Job drawing, mm, ordinate dimensions from the low corner. One solid piece. A direction names the side the tool comes from. Give positions to 0.01 mm unless a question says otherwise; leave off trailing zeros. Write each loop counter-clockwise with the first axis right and the second up, starting at its lowest first coordinate (ties: lowest second). Pieces come first, ordered by that corner, then holes. Notation, with made-up numbers: (-8.75, 83) - (44.25, 83) arc R36 ccw to (44.25, 122) - close; hole circle Ø10 at (0, -37.5). An arc over 180 degrees is marked (long way). Answer as a JSON object with one key per item and string values.
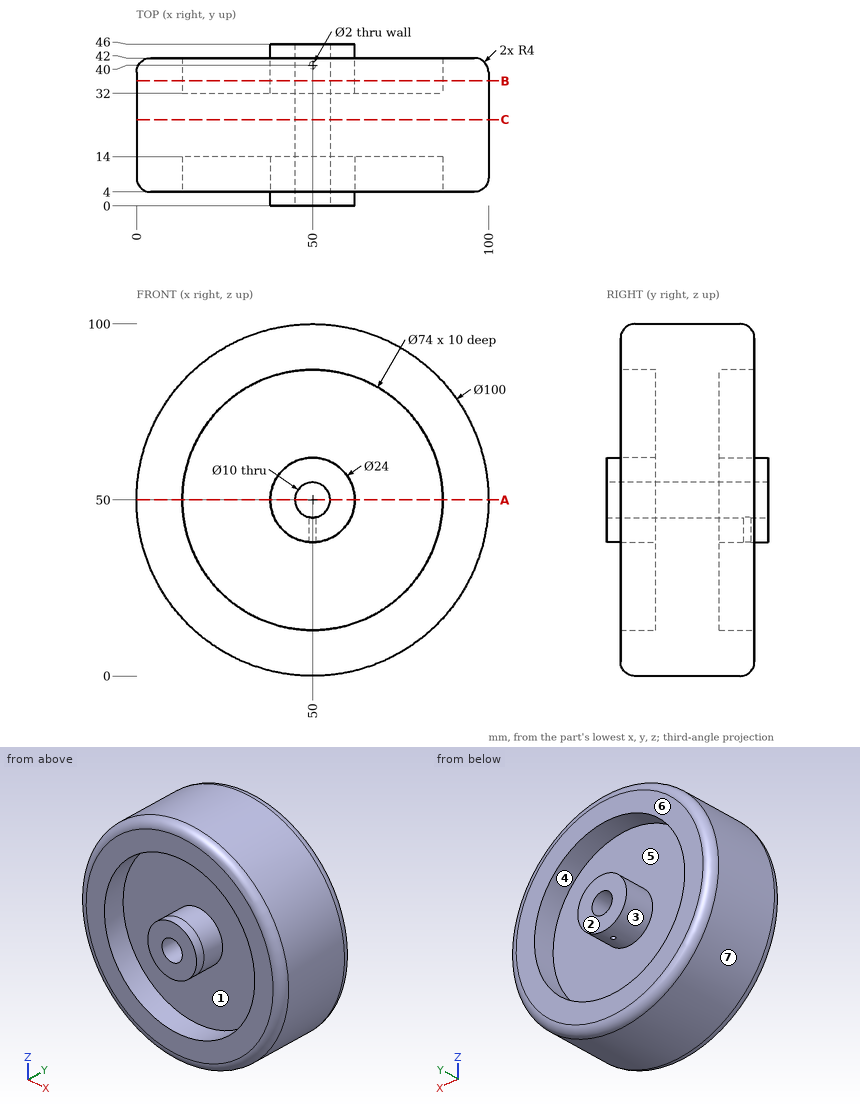
Item 1: Flat gauge pins, fed straight in: P1, Ø12, axis at x = 76.5, z = 62.5, coming from the -Y side; P2, Ø1.5, axis at x = 89, z = 57, coming from the -Y side; P3, Ø3, axis at x = 50, y = 40, coming from the -Z side. Where does each tip first touch, or does it go through?
Entries:
{"P1": "y = 14", "P2": "y = 4", "P3": "z = 0.03"}
Item 2: Probe line 1 (X direction, y = 8.5, z = 50); line 2 (Z direction, x = 53.5, y = 37.5); line 3 (X direction, y = 7, z = 50). List the from-to ranges inside material, lowest first. Write a range as from..to.
Entries:
{"line 1": "0..13, 38..45, 55..62, 87..100", "line 2": "0.12..13.17, 38.52..46.43, 53.57..61.48, 86.83..99.88", "line 3": "0.13..13, 38..45, 55..62, 87..99.87"}
Item 3: Mould opens along Z. For the marked faces 4, 5, 6 and 7 say: +Z half, -Z half, draft (parallel to the pull), parting line (faces both ways), or undercut.
Entries:
{"face 4": "undercut", "face 5": "undercut", "face 6": "draft", "face 7": "parting line"}
Item 4: Cut at B-B (y = 35.5). Give the cut face in (x, z), and give its area (3 significant figures).
Entries:
{"outline": "circle Ø100 at (50, 50); circle Ø24 at (50, 50); hole circle Ø74 at (50, 50); hole circle Ø10 at (50, 50)", "area": "3,930 mm2"}
Item 5: Cut at A-A (z = 50). Give the cut face in (x, y), and give its area (3 significant figures).
Entries:
{"outline": "(0, 8) arc R4 ccw to (4, 4) - (13, 4) - (13, 14) - (38, 14) - (38, 0) - (45, 0) - (45, 46) - (38, 46) - (38, 32) - (13, 32) - (13, 42) - (4, 42) arc R4 ccw to (0, 38) - close; (55, 0) - (62, 0) - (62, 14) - (87, 14) - (87, 4) - (96, 4) arc R4 ccw to (100, 8) - (100, 38) arc R4 ccw to (96, 42) - (87, 42) - (87, 32) - (62, 32) - (62, 46) - (55, 46) - close", "area": "2,520 mm2"}
Item 6: Which spindle directions (+Z, -Z, +X, -X, +Y, -Y) get a long thin tool onto all of the face, cutting with end or side? Do the marked faces 1, 2 and 3. Say none if no direction does.
Entries:
{"face 1": "-Y", "face 2": "+Z, -Z, +X, -X, +Y", "face 3": "+Y"}
Item 7: Cut at C-C (y = 24.5). Give the cut face in (x, z).
Entries:
{"outline": "circle Ø100 at (50, 50); hole circle Ø10 at (50, 50)"}
